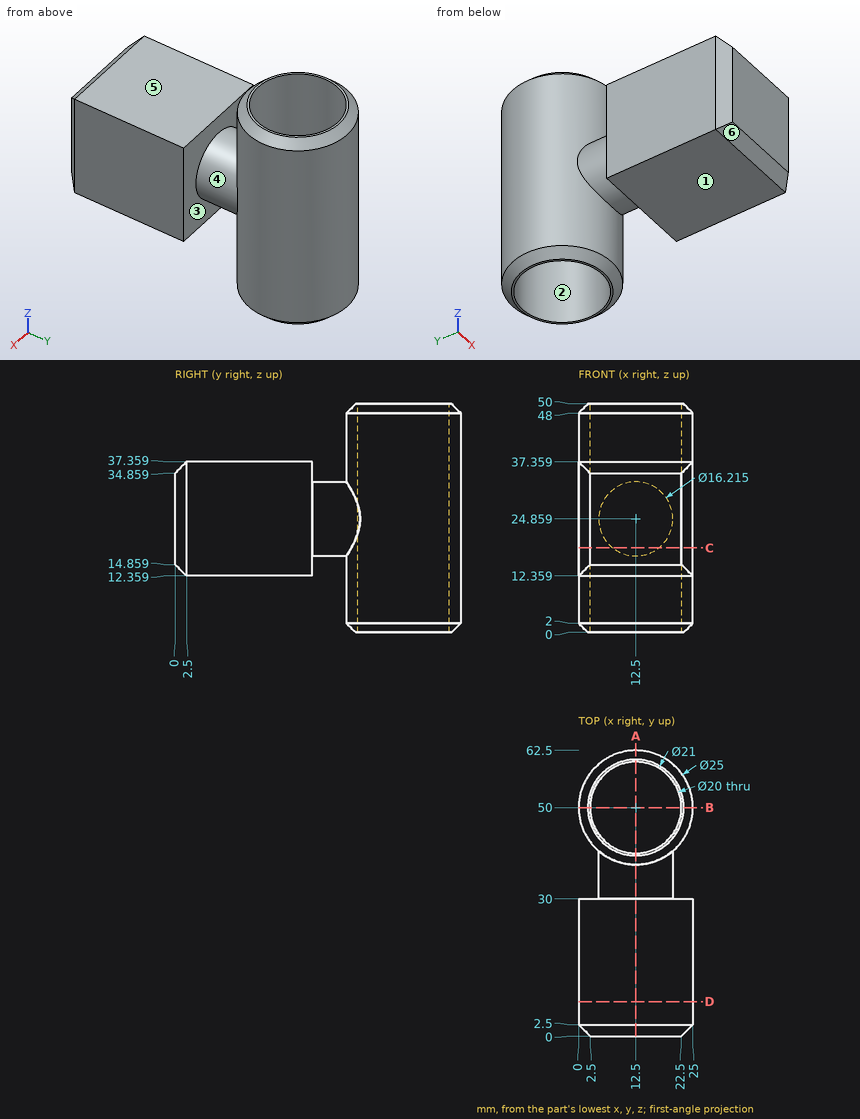
Could you check a few things on this drawing? It's one solid part, dimensions in mm from its lowest x, y, z. A direction names the side the tool comes from. Round coordinates to 2 decimals unless told otherwise and drop trailing zeros. Loops run counter-clockwise (first coordinate to the right, second up) from the corner with the lowest first, then second, coordinate; pieces in that order, holes last. Notation, with made-up numbers: (6.5, -25) -> (33.5, -25) arc R29 cw to (33.5, 2) -> close; hole circle Ø4 at (21.25, 68). An arc over 180 degrees is marked (long way). One line per item, written item: value. Start each with the question number.
1. If we section it at B-B, the plane y = 50: Write out the boundary of the cut face in (x, z), then the cut area to 3 significant figures.
2. For the marked faces 1, 2 and 3, which set-ups out of +Z, -Z, +X, -X, +Y, -Y let a thin tool reach every point of the face, with its end or its side?
3. If we section it at C-C, the plane z = 18.5: Write out the boundary of the cut face in (x, y).
4. If we section it at D-D, the plane y = 7.5: Write out the boundary of the cut face in (x, z), then the cut area to 3 significant figures.
5. For pin 1 (12 mm diameter, centred on x = 5, y = 25, fed in from +Z); pin 2 (1 mm diameter, centred on y = 41.5, z = 27, fed in from +X) (1 decimal); pin 3 (12 mm diameter, centred on x = 21.5, y = 12, fed in from -Z), each with a flat end and sliding along its axis, tell me the tip position at first contact or that it passes through.
6. If I drill on probe 1 along Y at (x, z) = (12, 10.5); probe 2 along Y at (x, z) = (19.75, 14) (1 decimal); probe 3 along Y at (x, z) = (13.5, 34), over which ranges is the centre line in solid material (lowest first)?
7. If we mould it in two halves opening along Y, with no side actions, what happens to the marked faces 4, 5 and 6? For each: pulls with the +Y half, pulls with the -Y half, needs draft (parallel to the pull), parting line crosses it, or undercut.
8. If we section it at A-A, the plane x = 12.5: Write out the boundary of the cut face in (y, z), then the cut area to 3 significant figures.
Calculated:
1. outline: (0, 2) -> (2, 0) -> (2.5, 0) -> (2.5, 50) -> (2, 50) -> (0, 48) -> close; (22.5, 0) -> (23, 0) -> (25, 2) -> (25, 48) -> (23, 50) -> (22.5, 50) -> close
1. area: 242 mm²
2. face 1: -Z, +X, -X, -Y
2. face 2: +Z, -Z
2. face 3: none
3. outline: (0, 2.5) -> (2.5, 0) -> (22.5, 0) -> (25, 2.5) -> (25, 30) -> (17.53, 30) -> (17.53, 38.56) arc R12.5 ccw (long way) to (7.47, 38.56) -> (7.47, 30) -> (0, 30) -> close; hole circle Ø20 at (12.5, 50)
4. outline: (0, 12.36) -> (25, 12.36) -> (25, 37.36) -> (0, 37.36) -> close
4. area: 625 mm²
5. pin 1: stops at z = 37.36
5. pin 2: stops at x = 22.1
5. pin 3: stops at z = 12.36
6. probe 1: y = 37.51 to 40.01, 59.99 to 62.49
6. probe 2: y = 0.9 to 30, 39.8 to 43.1, 56.9 to 60.2
6. probe 3: y = 0 to 30, 37.54 to 40.05, 59.95 to 62.46
7. face 4: undercut
7. face 5: needs draft
7. face 6: pulls with the -Y half
8. outline: (0, 14.86) -> (2.5, 12.36) -> (30, 12.36) -> (30, 16.75) -> (37.5, 16.75) -> (37.5, 2) -> (39.5, 0) -> (40, 0) -> (40, 50) -> (39.5, 50) -> (37.5, 48) -> (37.5, 32.97) -> (30, 32.97) -> (30, 37.36) -> (2.5, 37.36) -> (0, 34.86) -> close; (60, 0) -> (60.5, 0) -> (62.5, 2) -> (62.5, 48) -> (60.5, 50) -> (60, 50) -> close
8. area: 1,110 mm²
